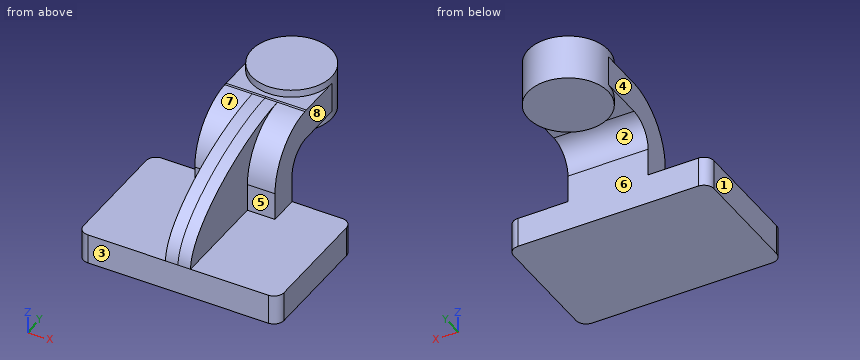
from build123d import *

# Parameters (mm, degrees)
F1_DEPTH = 63.5
F0_W     = 25.4
F0_H     = 19.05
F2_DEPTH = 25.4
F3_DEPTH = 7.9375
F5_R     = 6.35


with BuildPart() as f1:
    # F0 (on Right) → F1 (new body, symmetric)
    with BuildSketch(Plane.YZ):
        Polygon((-41.275, 9.525), (-41.275, -9.525), (41.275, -9.525), (41.275, 9.525), (22.225, 9.525), align=None)
    extrude(amount=F1_DEPTH, both=True)

    # F0 (on Right) → F2 (join, symmetric)
    with BuildSketch(Plane.YZ):
        with BuildLine():
            Line((22.225, 9.525), (41.275, 9.525))
            Line((41.275, 9.525), (41.275, 27.0002))
            ThreePointArc((41.275, 27.0002), (45.9246798487, 38.2255201513), (57.15, 42.8752))
            Line((57.15, 42.8752), (60.325, 42.8752))
            Line((60.325, 42.8752), (60.325, 61.9252))
            Line((60.325, 61.9252), (57.15, 61.9252))
            add(Edge.make_bspline(
                [(55.6725300952, 61.8939345046), (56.1670957389, 61.9078019398), (56.659625513, 61.9182367743), (57.15, 61.9252)],
                knots=[110.1817471717, 110.1817471717, 110.1817471717, 110.1817471717, 111.5045361635, 111.5045361635, 111.5045361635, 111.5045361635], degree=3))
            ThreePointArc((55.6725300952, 61.8939345046), (31.9373418555, 51.1678952622), (22.225, 27.0002))
            Line((22.225, 27.0002), (22.225, 9.525))
        make_face()
        with Locations((73.025, 52.4002)):
            Rectangle(F0_W, F0_H)
    extrude(amount=F2_DEPTH, both=True)

    # F0 (on Right) → F3 (join, symmetric)
    with BuildSketch(Plane.YZ):
        with BuildLine():
            add(Edge.make_bspline(
                [(-41.275, 9.525), (-40.8421786734, 35.7681623922), (14.4776705555, 60.7388460936), (55.6725300952, 61.8939345046)],
                knots=[0, 0, 0, 0, 110.1817471717, 110.1817471717, 110.1817471717, 110.1817471717], degree=3))
            Line((-41.275, 9.525), (22.225, 9.525))
            Line((22.225, 9.525), (22.225, 27.0002))
            ThreePointArc((22.225, 27.0002), (31.9373418555, 51.1678952622), (55.6725300952, 61.8939345046))
        make_face()
    extrude(amount=F3_DEPTH, both=True)

    # F0 (on Right) → F4 (revolve)
    with BuildSketch(Plane.YZ):
        Polygon((85.725, 66.675), (85.725, 61.9252), (85.725, 42.8752), (85.725, 38.1), (111.125, 38.1), (111.125, 66.675), align=None)
    revolve(axis=Axis((0, 85.725, 52.3875), (0, 0, 1)))

    # F5
    f5_edges = [f1.edges().sort_by_distance(p)[0] for p in [
        (63.5, 41.275, 0),
        (63.5, -41.275, 0),
        (-63.5, 41.275, 0),
        (-63.5, -41.275, 0),
    ]]
    fillet(f5_edges, radius=F5_R)


solid = f1.part
Verification items for the finished model (mm, model axes). Face numbers are marked on the shaded views. A direction names the side the tool comes from. Give positions to 0.01 mm unless a question says otherwise; leave off trailing zeros. Loops run counter-clockwise (first coordinate to the right, second up) from the corner with the lowest first, then second, coordinate; pieces in that order, holes last. Notation, with made-up numbers: (45.5, 16.5) - (78.5, 16.5) arc R24 cw to (78.5, 36.5) - close; hole circle Ø11 at (62.25, -8.5). An arc over 180 degrees is marked (long way). Write each question's results on one line, items separated by ' | '.
1) Mould release check, pull along Y, two halves, no side actions. Record for the marked faces 1, 2 and 3: pulls with the +Y half, pulls with the -Y half, needs draft (parallel to the pull), parting line crosses it, or undercut.
Solution:
face 1: needs draft | face 2: undercut | face 3: pulls with the -Y half
2) Material ranges on L1, parallel to Y at x = -21, z = 22 (3 decimals); L2, parallel to Y at x = 5.5, z = 1 (3 decimals); L3, parallel to Z at x = 30.5, y = 3 (3 decimals), recorded low to high. Write a range as from..to.
Solution:
L1: 22.225..41.275 | L2: -41.275..41.275 | L3: -9.525..9.525
3) Sectioned sample at B-B on y = 97.5. Record the boundary of the cut face in (x, z) (3 decimals), plus the area to 3 significant figures.
Solution:
outline: (-22.506, 38.1) - (22.506, 38.1) - (22.506, 66.675) - (-22.506, 66.675) - close | area: 1,290 mm2
4) Tool access check on the marked faces 4, 5, 6, 7 and 8. Record the directions out of +Z, -Z, +X, -X, +Y, -Y that give a thin tool (end or side, any length) a straight path to the whole face; none if there is none.
Solution:
face 4: +Z, -X, +Y, -Y | face 5: +Z, +X, -Y | face 6: -Z, +X, -X, +Y | face 7: +Z, -X, -Y | face 8: +Z, +X, +Y, -Y
5) Depth check by flat-ended pin: P1, Ø1.5, axis at x = -1, z = 36, coming from the +Y side; P2, Ø5, axis at x = 43, z = 5, coming from the +Y side (3 decimals); P3, Ø15, axis at x = -9, y = 75, coming from the -Z side. Enter the tip coordinate at first touch or a pass-through.
Solution:
P1: y = 44.62 | P2: y = 41.275 | P3: z = 38.1
6) Sectioned sample at A-A on x = -38.5. Record the boundary of the cut face in (y, z) (3 decimals), plus the area to 3 significant figures.
Solution:
outline: (-41.275, -9.525) - (41.275, -9.525) - (41.275, 9.525) - (-41.275, 9.525) - close | area: 1,570 mm2
